Here's how the part is built. I have some questions about the finished solid (model axes, mm). A direction names the side the tool comes from. Coordinates: 2 decimals unless noted, no trailing zeros. Write each loop counter-clockwise with the first axis right and the second up, starting at its lowest first coordinate (ties: lowest second). Pieces come first, ordered by that corner, then holes.
Item 1: If we section it at A-A (y = 7.65): Please give me the cut outline in (x, z), then the cut area to 3 significant figures.
Item 2: For faces 1 (the face through (-3.4, 0, 3)), 2 (the face through (4.31, 5.25, 0.62)), 3 (the face through (0.1, 5.3, 4.3)), which set-ups out of +Z, -Z, +X, -X, +Y, -Y let a thin tool reach every point of the face, with its end or its side?
Item 3: I'm going to push flat-ended pins straight in: pin 1 Ø1.4 at (y, z) = (10, -3.5) entering from +X; pin 2 Ø1 at (x, y) = (2, 4) entering from -Z; pin 3 Ø0.8 at (x, z) = (0, -8.7) entering from +Y; pin 4 Ø0.8 at (x, z) = (0, -7.5) entering from -Y. Where does each tip first touch, or does it pass through?
Item 4: If I drill on line 1 (Z direction, x = 0, y = 11); line 2 (Z direction, x = 4.85, y = 7.65); line 3 (Z direction, x = -3.5, y = -2.5), over which ranges is the centre line in solid material (lowest first)?
Item 5: If we section it at B-B (y = 3.25): Please give me the cut outline in (x, z), then the cut area to 3 significant figures.
Item 6: We'd pull the mould along Z, two halves only. Please class faces 4 (the face through (0.152, 10.847, -9.383)), 5 (the face through (-4.5, 4, -2)), 6 (the face through (4.7, 7.6, -10.1)): +Z half, -Z half, draft (parallel to the pull), parting line (faces both ways), or undercut.
Item 7: If we section it at D-D (x = 2.25): Please give me the cut outline in (y, z).
Item 8: If we section it at C-C (z = -0.5): Please give me the cut outline in (x, y).
from build123d import *

# Parameters (mm, degrees)
F1_DEPTH  = 10.65
F2_W      = 9
F2_H      = 10.7
F3_DEPTH  = 3.5
F4_R      = 1
F5_R      = 0.7
F6_DEPTH  = 0.4
F7_R      = 0.7
F8_DEPTH  = 0.4
F10_R     = 0.7
F11_DEPTH = 0.05


with BuildPart() as f1:
    # F0 (on Front) → F1 (new body)
    with BuildSketch(Plane.XZ):
        with BuildLine():
            ThreePointArc((4.1088888889, 1.2676876976), (0, 4.3), (-4.1088888889, 1.2676876976))
            Line((-4.1088888889, 1.2676876976), (-4.5, 0))
            Line((-4.5, 0), (-4.5, -6.4))
            Line((-4.5, -6.4), (0, -6.4))
            Line((0, -6.4), (4.5, -6.4))
            Line((4.5, -6.4), (4.5, 0))
            Line((4.5, 0), (4.1088888889, 1.2676876976))
        make_face()
    extrude(amount=-F1_DEPTH)

    # F2 (on face) → F3 (join)
    with BuildSketch(Plane.XZ):
        with Locations((0, -1.05)):
            Rectangle(F2_W, F2_H)
    extrude(amount=F3_DEPTH)

    # F4
    f4_edges = [f1.edges().sort_by_distance(p)[0] for p in [
        (4.5, -1.75, 4.3),
        (-4.5, -1.75, 4.3),
        (4.5, 3.575, -6.4),
        (-4.5, 3.575, -6.4),
    ]]
    fillet(f4_edges, radius=F4_R)

    # F5 (on face) → F6 (join)
    with BuildSketch(Plane.YZ.offset(4.5)):
        with BuildLine():
            ThreePointArc((6.45, -8.9), (7.65, -10.1), (8.85, -8.9))
            Line((8.85, -8.9), (8.85, 0))
            Line((8.85, 0), (6.45, 0))
            Line((6.45, 0), (6.45, -8.9))
        make_face()
        with Locations((7.65, -8.9)):
            Circle(F5_R, mode=Mode.SUBTRACT)
    extrude(amount=F6_DEPTH)

    # F7 (on face) → F8 (join)
    with BuildSketch(Plane(origin=(0, 10.65, 0), x_dir=(-1, 0, 0), z_dir=(0, 1, 0))):
        with BuildLine():
            ThreePointArc((-1.4, -8.7), (0, -10.1), (1.4, -8.7))
            Line((1.4, -8.7), (1.4, 0))
            Line((1.4, 0), (-1.4, 0))
            Line((-1.4, 0), (-1.4, -8.7))
        make_face()
        with Locations((0, -8.7)):
            Circle(F7_R, mode=Mode.SUBTRACT)
    extrude(amount=F8_DEPTH)

    # F10 (on offset) → F11 (join, symmetric)
    with BuildSketch(Plane.XZ.offset(-4.05)):
        with BuildLine():
            ThreePointArc((-1.25, -8.7), (0, -9.95), (1.25, -8.7))
            Line((1.25, -8.7), (1.25, 0))
            Line((1.25, 0), (-1.25, 0))
            Line((-1.25, 0), (-1.25, -8.7))
        make_face()
        with Locations((0, -8.7)):
            Circle(F10_R, mode=Mode.SUBTRACT)
    extrude(amount=F11_DEPTH, both=True)


solid = f1.part
Answer list:
1. outline: (-4.5, -5.4) arc R1 ccw to (-3.5, -6.4) - (3.5, -6.4) arc R1 ccw to (4.5, -5.4) - (4.5, -8.2) - (4.9, -8.2) - (4.9, 0) - (4.5, 0) - (4.11, 1.27) arc R4.3 ccw to (-4.11, 1.27) - (-4.5, 0) - close; (4.5, -10.1) - (4.9, -10.1) - (4.9, -9.6) - (4.5, -9.6) - close
1. area: 89.9 mm2
2. face 1: +Z, -X, +Y
2. face 2: +Z, +X, +Y
2. face 3: +Z, +Y
3. pin 1: stops at x = 4.5
3. pin 2: stops at z = -6.4
3. pin 3: passes through
3. pin 4: stops at y = 4
4. line 1: z = -10.1 to -9.4, -8 to 0
4. line 2: z = -10.1 to -9.6, -8.2 to 0
4. line 3: z = -6.4 to 4.3
5. outline: (-4.5, -5.4) arc R1 ccw to (-3.5, -6.4) - (3.5, -6.4) arc R1 ccw to (4.5, -5.4) - (4.5, 0) - (4.11, 1.27) arc R4.3 ccw to (-4.11, 1.27) - (-4.5, 0) - close
5. area: 86.4 mm2
6. face 4: undercut
6. face 5: draft
6. face 6: -Z half
7. outline: (-3.5, -6.4) - (10.65, -6.4) - (10.65, 3.66) - (0, 3.66) - (0, 4.3) - (-3.5, 4.3) - close
8. outline: (-4.5, -3.5) - (4.5, -3.5) - (4.5, 6.45) - (4.9, 6.45) - (4.9, 8.85) - (4.5, 8.85) - (4.5, 10.65) - (1.4, 10.65) - (1.4, 11.05) - (-1.4, 11.05) - (-1.4, 10.65) - (-4.5, 10.65) - close
